Check sheet for the drawn part. Datum: minimum x, y, z corner. Units: mm. A direction names the side the tool comes from. Round coordinates to 2 decimals unless told otherwise and drop trailing zeros. Write each loop counter-clockwise with the first axis right and the second up, starting at its lowest first coordinate (ties: lowest second). Pieces come first, ordered by that corner, then holes. Notation, with made-up numbers: M 78.25,74 L 119.25,74 A21 ccw 119.25,91 Z; hole C 49.5,-21.5 d7. An arc over 180 degrees is marked long. One line per item, written item: value. Start each with the question number.
1. Section check A-A (x = 10). Record the boundary of the cut face in (y, z), and give its area (3 significant figures).
2. Section check B-B (z = 10.5). Record the boundary of the cut face in (x, y).
3. Depth check by flat-ended pin: P1, Ø1.5, axis at x = 3.5, y = 12.5, coming from the +Z side; P2, Ø2, axis at x = 11.5, z = 3.5, coming from the +Y side; P3, Ø5, axis at x = 5, z = 9.5, coming from the -Y side. Enter the tip coordinate at first touch or a pass-through.
4. Access from +Z, -Z, +X, -X, +Y, -Y to the whole of each face (thin tool, end or side, straight path). Record for the marked faces 1, 2 and 3.
5. Scan lines: probe 1 along Z at (x, y) = (11.75, 13.75); probe 2 along X at (y, z) = (10, 16); probe 3 along Y at (x, z) = (7, 10.5). Record each from-to range of solid material in increasing order. Write a range as [from, to].
6. Section check C-C (y = 8.25). Record the boundary of the cut face in (x, z), and give its area (3 significant figures).
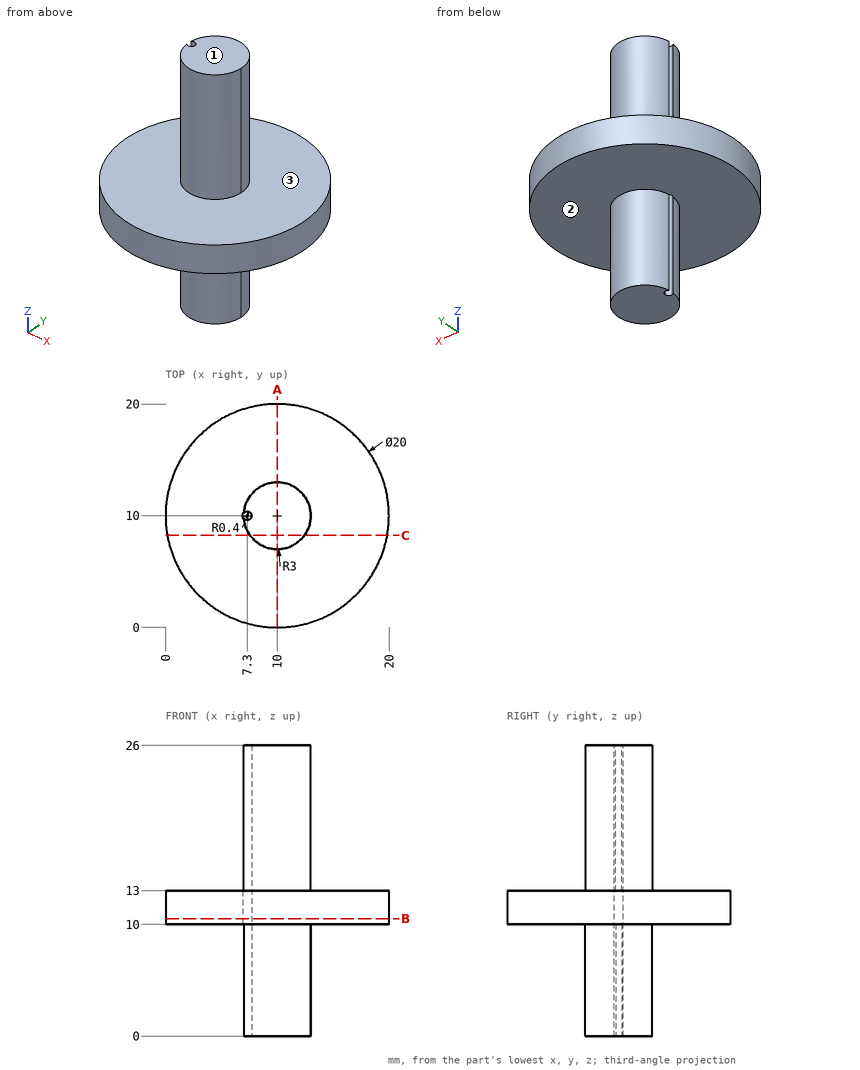
Result sheet:
1. outline: M 0,10 L 7,10 L 7,0 L 13,0 L 13,10 L 20,10 L 20,13 L 13,13 L 13,26 L 7,26 L 7,13 L 0,13 Z
1. area: 198 mm2
2. outline: C 10,10 d20; hole C 7.3,10 d0.8
3. P1: stops at z = 13
3. P2: stops at y = 12.96
3. P3: stops at y = 0.33
4. face 1: +Z, +X, -X, +Y, -Y
4. face 2: -Z
4. face 3: +Z
5. probe 1: z = [10, 13]
5. probe 2: x = [7.7, 13]
5. probe 3: y = [0.46, 9.74], [10.26, 19.54]
6. outline: M 0.15,10 L 7.56,10 L 7.56,0 L 12.44,0 L 12.44,10 L 19.85,10 L 19.85,13 L 12.44,13 L 12.44,26 L 7.56,26 L 7.56,13 L 0.15,13 Z
6. area: 171 mm2
